```python
from build123d import *

# Parameters (mm, degrees)
SKETCH1_R           = 55
BOSS_EXTRUDE1_DEPTH = 17
SKETCH2_R           = 15
CUT_EXTRUDE1_DEPTH  = 80.617837197
SKETCH3_R           = 3.964920539
CUT_EXTRUDE2_DEPTH  = 14.720649
CIRPATTERN1_START   = 2.279350926
CIRPATTERN1_DEPTH   = 14.720649074


# Read off the part's stored shape, not the designer's step: CirPattern1
with BuildPart() as part:
    # Sketch1 → Boss-Extrude1 (new body)
    with BuildSketch(Plane(origin=(0, 0, 0), x_dir=(1, 0, 0), z_dir=(0, 1, 0))):
        with Locations(Location((0, 0, 0), (0, 0, 270))):
            Circle(SKETCH1_R)
    extrude(amount=BOSS_EXTRUDE1_DEPTH)

    # Sketch2 → Cut-Extrude1 (cut, through all)
    with BuildSketch(Plane(origin=(0, 0, 0), x_dir=(1, 0, 0), z_dir=(0, 1, 0))):
        with Locations(Location((0, 0, 0), (0, 0, 270))):
            Circle(SKETCH2_R)
    extrude(amount=CUT_EXTRUDE1_DEPTH, mode=Mode.SUBTRACT)

    # Sketch3 → Cut-Extrude2 (cut)
    with BuildSketch(Plane(origin=(0, 17, 0), x_dir=(1, 0, 0), z_dir=(0, 1, 0))):
        with Locations((-17.758888816, 0)):
            Circle(SKETCH3_R)
    extrude(amount=-CUT_EXTRUDE2_DEPTH, mode=Mode.SUBTRACT)

    # CirPattern1 outline → CirPattern1 (cut)
    with BuildSketch(Plane(origin=(0, 0, 0), x_dir=(1, 0, 0), z_dir=(0, 1, 0)).offset(CIRPATTERN1_START)):
        with BuildLine():
            ThreePointArc((-2.60714929, 14.77168821), (0, 15), (2.60714929, 14.77168821))
            ThreePointArc((2.60714929, 14.77168821), (0, 21.723809355), (-2.60714929, 14.77168821))
        make_face()
        with BuildLine():
            ThreePointArc((14.77168821, -2.60714929), (21.723809355, 0), (14.77168821, 2.60714929))
            ThreePointArc((14.77168821, 2.60714929), (15, 0), (14.77168821, -2.60714929))
        make_face()
        with BuildLine():
            ThreePointArc((2.60714929, -14.77168821), (0, -15), (-2.60714929, -14.77168821))
            ThreePointArc((-2.60714929, -14.77168821), (0, -21.723809355), (2.60714929, -14.77168821))
        make_face()
    extrude(amount=CIRPATTERN1_DEPTH, mode=Mode.SUBTRACT)


solid = part.part
```
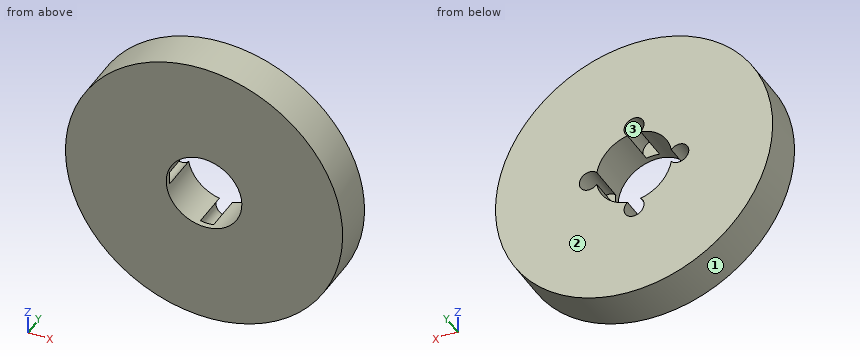
Design review of the part built by this model. Coordinates are the model's own, in mm. Face numbers are marked on the shaded views. Give positions to 0.01 mm unless a question says otherwise; leave off trailing zeros. Write each loop counter-clockwise with the first axis right and the second up, starting at its lowest first coordinate (ties: lowest second). Pieces come first, ordered by that corner, then holes. Notation, with made-up numbers: (70, -13.75) -> (90, -13.75) arc R9 ccw to (90, -5.75) -> close; hole circle Ø7 at (41, -6). An arc over 180 degrees is marked (long way). Answer in a Markdown table with one row per item.
(1) Consider section D-D (x = 20). State the section outline as (y, z) points, then the cut area to 3 significant figures.
Results:
| item | result |
|---|---|
| outline | (0, -51.23) -> (17, -51.23) -> (17, -3.27) -> (2.28, -3.27) -> (2.28, 3.27) -> (17, 3.27) -> (17, 51.23) -> (0, 51.23) -> close |
| area | 1,650 mm2 |
(2) To check wall thickness, follow probe 1 along Z at (x, y) = (8, 16.25); probe 2 along X at (y, z) = (12.75, -19.5); probe 3 along Z at (x, y) = (-8.5, 4.25). State the ranges of each line that lie inside material, in increasing order.
Results:
| item | result |
|---|---|
| probe 1 | -54.42 to -12.69, 12.69 to 54.42 |
| probe 2 | -51.43 to -3.56, 3.56 to 51.43 |
| probe 3 | -54.34 to -12.36, 12.36 to 54.34 |
(3) Consider section C-C (y = 15). State the section outline as (x, z) points, then the cut area to 3 significant figures.
Results:
| item | result |
|---|---|
| outline | circle Ø110 at (0, 0); hole (-14.77, -2.61) arc R15 ccw to (-2.61, -14.77) arc R3.96 ccw (long way) to (2.61, -14.77) arc R15 ccw to (14.77, -2.61) arc R3.96 ccw (long way) to (14.77, 2.61) arc R15 ccw to (2.61, 14.77) arc R3.96 ccw (long way) to (-2.61, 14.77) arc R15 ccw to (-14.77, 2.61) arc R3.96 ccw (long way) to start |
| area | 8,620 mm2 |
(4) Mouldability with a two-part tool opening along Z and no side actions: class the marked faces 1, 2 and 3 as +Z half, -Z half, draft (parallel to the pull), parting line (faces both ways), or undercut.
Results:
| item | result |
|---|---|
| face 1 | parting line |
| face 2 | draft |
| face 3 | undercut |
(5) Consider section B-B (x = 0). State the section outline as (y, z) points.
Results:
| item | result |
|---|---|
| outline | (0, -55) -> (17, -55) -> (17, -21.72) -> (2.28, -21.72) -> (2.28, -15) -> (0, -15) -> close; (0, 15) -> (2.28, 15) -> (2.28, 21.72) -> (17, 21.72) -> (17, 55) -> (0, 55) -> close |
(6) Clearance check with flat-ended pins moving along their axes: pin 1 (3 mm diameter, centred on y = 6, z = -8, fed in from -X); pin 2 (2 mm diameter, centred on x = 0.5, z = -19.5, fed in from +Y); pin 3 (12.5 mm diameter, centred on x = 17.76, z = 0, fed in from +Y); pin 4 (1 mm diameter, centred on y = 2.5, z = 33.5, fed in from -X). State where each tip first meets the part, or that it passes through.
Results:
| item | result |
|---|---|
| pin 1 | x = -54.61 |
| pin 2 | y = 2.28 |
| pin 3 | y = 17 |
| pin 4 | x = -44 |
(7) Consider section A-A (z = 0). State the section outline as (x, y) points, then the cut area to 3 significant figures.
Results:
| item | result |
|---|---|
| outline | (-55, 0) -> (-15, 0) -> (-15, 2.28) -> (-21.72, 2.28) -> (-21.72, 17) -> (-55, 17) -> close; (15, 0) -> (55, 0) -> (55, 17) -> (21.72, 17) -> (21.72, 2.28) -> (15, 2.28) -> close |
| area | 1,160 mm2 |
